Source: CAD feature listing. Evaluate the final solid. Frame: model axes, mm. Round coordinates to 2 decimals unless told otherwise and drop trailing zeros. Write each loop counter-clockwise with the first axis right and the second up, starting at its lowest first coordinate (ties: lowest second). Pieces come first, ordered by that corner, then holes. Notation, with made-up numbers: M 26.25,29.25 L 55.25,29.25 A16 cw 55.25,43.25 Z; hole C 22,-3 d7. An arc over 180 degrees is marked long. Put each result on its own line as item: value. Start each with the question number.
```python
from build123d import *

# Parameters (mm, degrees)
SKETCH1_R           = 1.25
SKETCH1_R_2         = 1.6
BOSS_EXTRUDE1_DEPTH = 1.5


with BuildPart() as part:
    # Sketch1 → Boss-Extrude1 (new body)
    with BuildSketch(Plane(origin=(0, 0, 0), x_dir=(1, 0, 0), z_dir=(0, 1, 0))):
        Polygon((57, 0), (57, 10), (55.4, 10), (55.4, 51.5), (57, 51.5), (57, 61.5), (55.4, 61.5), (55.4, 103), (57, 103), (57, 113), (47, 113), (47, 111.4), (33.5, 111.4), (33.5, 113), (23.5, 113), (23.5, 111.4), (10, 111.4), (10, 113), (0, 113), (0, 103), (1.6, 103), (1.6, 61.5), (0, 61.5), (0, 51.5), (1.6, 51.5), (1.6, 10), (0, 10), (0, 0), (10, 0), (10, 1.6), (23.5, 1.6), (23.5, 0), (33.5, 0), (33.5, 1.6), (47, 1.6), (47, 0), align=None)
        with Locations((20.88, 108.8)):
            Circle(SKETCH1_R, mode=Mode.SUBTRACT)
        with Locations((36.12, 108.8)):
            Circle(SKETCH1_R, mode=Mode.SUBTRACT)
        with Locations((20, 77.964629758)):
            Circle(SKETCH1_R_2, mode=Mode.SUBTRACT)
        with Locations((37, 77.964629758)):
            Circle(SKETCH1_R_2, mode=Mode.SUBTRACT)
        with Locations((20, 21.964629758)):
            Circle(SKETCH1_R_2, mode=Mode.SUBTRACT)
        with Locations((37, 21.964629758)):
            Circle(SKETCH1_R_2, mode=Mode.SUBTRACT)
    extrude(amount=BOSS_EXTRUDE1_DEPTH)


solid = part.part
```
(1) Section query B-B (y = 0.95). Count the separate pieces of the cut face and the enclosed holes in it, and give its area (3 significant figures).
(2) Pull-direction query (X, two-part tool) for faces 1 (the flat face through (28, 1.5, -57)), 2 (the cylindrical face through (21.457, 0.74, -107.691)); classes: +X half, -X half, draft (parallel to the pull), parting line (faces both ways), or undercut.
(3) Ray query, line 1 along Z through (x, y) = (37, 0.95); line 2 along X through (y, z) = (1.05, -108.8); line 3 along X through (y, z) = (0.4, -21). Return the intervals inside material, ascending.
(4) Section query A-A (z = -108.8). Return loops of the section in (x, y).
Entries:
1. separate pieces: 1
1. enclosed holes: 6
1. area: 6,050 mm2
2. face 1: draft
2. face 2: undercut
3. line 1: -111.4 to -109.69, -107.91 to -79.56, -76.36 to -23.56, -20.36 to -1.6
3. line 2: 0 to 19.63, 22.13 to 34.87, 37.37 to 57
3. line 3: 1.6 to 18.72, 21.28 to 35.72, 38.28 to 55.4
4. outline: M 0,0 L 19.63,0 L 19.63,1.5 L 0,1.5 Z; M 22.13,0 L 34.87,0 L 34.87,1.5 L 22.13,1.5 Z; M 37.37,0 L 57,0 L 57,1.5 L 37.37,1.5 Z
